```python
from build123d import *

# Parameters (mm, degrees)
SKETCH1_W           = 101.6
SKETCH1_H           = 37
BOSS_EXTRUDE1_DEPTH = 5.334
SKETCH2_R           = 15.5
MOTOR_HOLE_DEPTH    = 55.326251076
SKETCH4_W           = 19.05
SKETCH4_H           = 5.334
BOTTOM_TABS_DEPTH   = 5.334
SKETCH5_W           = 5.334
SKETCH5_H           = 12.7
CUT_EXTRUDE1_DEPTH  = 57.366223148
SKETCH6_W           = 15.24
SKETCH6_H           = 12.7
CUT_EXTRUDE2_DEPTH  = 77.262693919


with BuildPart() as part:
    # Sketch1 → Boss-Extrude1 (new body)
    with BuildSketch(Plane.XY):
        Rectangle(SKETCH1_W, SKETCH1_H)
    extrude(amount=-BOSS_EXTRUDE1_DEPTH)

    # Sketch2 → Motor Hole (cut, through all)
    with BuildSketch(Plane.XY):
        Circle(SKETCH2_R)
    extrude(amount=-MOTOR_HOLE_DEPTH, mode=Mode.SUBTRACT)

    # Sketch4 → Bottom Tabs (add)
    with BuildSketch(Plane.XZ.offset(18.5)):
        with Locations((-41.275, -2.667)):
            Rectangle(SKETCH4_W, SKETCH4_H)
        with Locations((0, -2.667)):
            Rectangle(SKETCH4_W, SKETCH4_H)
        with Locations((41.275, -2.667)):
            Rectangle(SKETCH4_W, SKETCH4_H)
    extrude(amount=BOTTOM_TABS_DEPTH)

    # Sketch5 → Cut-Extrude1 (cut, through all)
    with BuildSketch(Plane.XY):
        with Locations((-48.133, 0)):
            Rectangle(SKETCH5_W, SKETCH5_H)
        with Locations((48.133, 0)):
            Rectangle(SKETCH5_W, SKETCH5_H)
    extrude(amount=-CUT_EXTRUDE1_DEPTH, mode=Mode.SUBTRACT)

    # Sketch6 → Cut-Extrude2 (cut, through all)
    with BuildSketch(Plane(origin=(16.243120564, -7.106483242, 20.4638), x_dir=(1, 0, 0), z_dir=(0, 0, 1))):
        with Locations((15.252879436, 0.290483242)):
            Rectangle(SKETCH6_W, SKETCH6_H)
    extrude(amount=-CUT_EXTRUDE2_DEPTH, mode=Mode.SUBTRACT)


solid = part.part
```
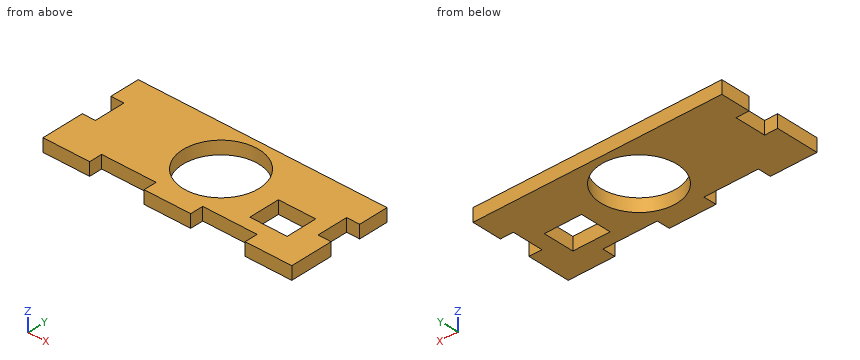
The listing builds one solid part. Answer for the finished solid, in the listing's coordinates (mm). Coordinates: 2 decimals unless noted, no trailing zeros. Loops run counter-clockwise (first coordinate to the right, second up) from the corner with the lowest first, then second, coordinate; pieces in that order, holes last. Notation, with made-up numbers: (-31.75, -17) -> (-14.75, -17) arc R37 ccw to (-14.75, 21) -> close; hole circle Ø6 at (15.5, 76.5). An arc over 180 degrees is marked (long way). Return JSON: item names as keys, results as strings. Group by question number.
(1) Given pin 1 Ø1.6 at (x, z) = (-22, -3.5) entering from -Y; pin 2 Ø3 at (y, z) = (4.5, -1) entering from +X, each flat-ended and moving along its own axis, determine where each tip first touches the part or whether it passes through.
(2) A cutting plane is placed at D-D on y = 8. Write down the section's boundary in (x, z).
(3) A cutting plane is placed at A-A on y = -21. Write down the section's boundary in (x, z) (3 decimals).
(4) A cutting plane is placed at B-B on z = -4.25. Write down the section's boundary in (x, y) (3 decimals).
(5) A cutting plane is placed at C-C on x = 0. Write down the section's boundary in (y, z).
(6) Find the intervals of material crossed by probe 1 along Y at (x, z) = (0, -1.7); probe 2 along X at (y, z) = (-10, -3.7); probe 3 along Y at (x, z) = (24.5, -5), in increasing order. Write a range as from..to.
The answers:
{
 "1": {"pin 1": "stops at y = -18.5", "pin 2": "stops at x = 45.47"},
 "2": {"outline": "(-50.8, -5.33) -> (-13.28, -5.33) -> (-13.28, 0) -> (-50.8, 0) -> close; (13.28, -5.33) -> (50.8, -5.33) -> (50.8, 0) -> (13.28, 0) -> close"},
 "3": {"outline": "(-50.8, -5.334) -> (-31.75, -5.334) -> (-31.75, 0) -> (-50.8, 0) -> close; (-9.525, -5.334) -> (9.525, -5.334) -> (9.525, 0) -> (-9.525, 0) -> close; (31.75, -5.334) -> (50.8, -5.334) -> (50.8, 0) -> (31.75, 0) -> close"},
 "4": {"outline": "(-50.8, -23.834) -> (-31.75, -23.834) -> (-31.75, -18.5) -> (-9.525, -18.5) -> (-9.525, -23.834) -> (9.525, -23.834) -> (9.525, -18.5) -> (31.75, -18.5) -> (31.75, -23.834) -> (50.8, -23.834) -> (50.8, -6.35) -> (45.466, -6.35) -> (45.466, 6.35) -> (50.8, 6.35) -> (50.8, 18.5) -> (-50.8, 18.5) -> (-50.8, 6.35) -> (-45.466, 6.35) -> (-45.466, -6.35) -> (-50.8, -6.35) -> close; hole circle Ø31 at (0, 0); hole (23.876, -13.166) -> (39.116, -13.166) -> (39.116, -0.466) -> (23.876, -0.466) -> close"},
 "5": {"outline": "(-23.83, -5.33) -> (-15.5, -5.33) -> (-15.5, 0) -> (-23.83, 0) -> close; (15.5, -5.33) -> (18.5, -5.33) -> (18.5, 0) -> (15.5, 0) -> close"},
 "6": {"probe 1": "y = -23.83..-15.5, 15.5..18.5", "probe 2": "x = -50.8..-11.84, 11.84..23.88, 39.12..50.8", "probe 3": "y = -18.5..-13.17, -0.47..18.5"}
}
